Can you work these out from the model? Positions are in its coordinate system, mm. Face numbers are marked on the shaded views. A direction names the side the tool comes from. Round coordinates to 2 decimals unless told otherwise and drop trailing zeros. Write each loop counter-clockwise with the first axis right and the second up, starting at its lowest first coordinate (ties: lowest second). Pieces come first, ordered by that corner, then holes.
Q1. For the marked faces 4, 5 and 6, which set-ups out of +Z, -Z, +X, -X, +Y, -Y let a thin tool reach every point of the face, with its end or its side?
Q2. If we section it at B-B (z = 15): Please give me the cut outline in (x, y), plus the area to 3 significant figures.
Q3. If we section it at D-D (x = -14.9): Please give me the cut outline in (y, z).
Q4. Please list where these lines run through material, in increasing order: line 1 along Y through (x, z) = (0.5, 25); line 2 along Y through (x, z) = (25, 8); line 3 along Y through (x, z) = (25.5, 6).
Q5. We'd pull the mould along X, two halves only. Please class the marked faces 1, 2 and 3: +X half, -X half, draft (parallel to the pull), parting line (faces both ways), or undercut.
Q6. If we section it at C-C (y = 0): Please give me the cut outline in (x, z).
Q7. If we section it at A-A (y = -5): Please give me the cut outline in (x, z).
Q8. I'm going to push flat-ended pins straight in: pin 1 Ø22.5 at (x, z) = (10.5, 11) entering from -Y; pin 2 Ø1 at (y, z) = (-11.5, 19.5) entering from -X; pin 3 Ø2.5 at (x, y) = (11.5, 1) entering from +Z. Where does each tip first touch, or does it pass through?
from build123d import *

# Parameters (mm, degrees)
SKETCH1_W                    = 49.7
SKETCH1_H                    = 26
BOSS_EXTRUDE1_DEPTH          = 14
SKETCH2_W                    = 41.4
SKETCH2_H                    = 26
BOSS_EXTRUDE2_DEPTH          = 17
CUT_EXTRUDE1_DEPTH           = 20.5
SKETCH4_W                    = 14
SKETCH4_H                    = 26
BOSS_EXTRUDE3_DEPTH          = 7.7
BOSS_EXTRUDE5_START          = -26
SKETCH6_W                    = 8
SKETCH6_H                    = 5
BOSS_EXTRUDE5_DEPTH          = 7
SKETCH5_W                    = 7
SKETCH5_H                    = 7
BOSS_EXTRUDE6_DEPTH          = 7
SKETCH7_W                    = 4
SKETCH7_H                    = 6.5
F_3_0_3_DIAMETER_HOLE1_D     = 3
F_3_0_3_DIAMETER_HOLE1_DEPTH = 38
F_3_0_3_DIAMETER_HOLE2_D     = 3
F_3_0_3_DIAMETER_HOLE2_DEPTH = 39.1
F_3_0_3_DIAMETER_HOLE3_D     = 3
F_3_0_3_DIAMETER_HOLE3_DEPTH = 33
FILLET1_R                    = 6


with BuildPart() as part:
    # Sketch1 → Boss-Extrude1 (new body)
    with BuildSketch(Plane(origin=(0, 0, 0), x_dir=(-1, 0, 0), z_dir=(0, 0, -1))):
        with Locations((3.85, 0)):
            Rectangle(SKETCH1_W, SKETCH1_H)
    extrude(amount=-BOSS_EXTRUDE1_DEPTH)

    # Sketch2 → Boss-Extrude2 (add)
    with BuildSketch(Plane.XY.offset(14)):
        Rectangle(SKETCH2_W, SKETCH2_H)
    extrude(amount=BOSS_EXTRUDE2_DEPTH)

    # Sketch3 → Cut-Extrude1 (cut)
    with BuildSketch(Plane(origin=(0, 10.25, 0), x_dir=(1, 0, 0), z_dir=(0, 1, 0))):
        Polygon((20.7, -14), (21, -14), (21, 0), (-21, 0), (-21, -14), (-20.7, -14), (-20.7, -28.1), (20.7, -28.1), align=None)
    extrude(amount=-CUT_EXTRUDE1_DEPTH, mode=Mode.SUBTRACT)

    # Sketch4 → Boss-Extrude3 (add)
    with BuildSketch(Plane(origin=(21, 0, 0), x_dir=(0, 0, -1), z_dir=(1, 0, 0))):
        with Locations((-7, 0)):
            Rectangle(SKETCH4_W, SKETCH4_H)
    extrude(amount=BOSS_EXTRUDE3_DEPTH)

    # Sketch6 → Boss-Extrude5 (add)
    with BuildSketch(Plane(origin=(0, 13, 0), x_dir=(-1, 0, 0), z_dir=(0, 1, 0)).offset(BOSS_EXTRUDE5_START)):
        with Locations((6.4, 2.5)):
            Rectangle(SKETCH6_W, SKETCH6_H)
    extrude(amount=-BOSS_EXTRUDE5_DEPTH)

    # Sketch5 → Boss-Extrude6 (add)
    with BuildSketch(Plane.XY.offset(31)):
        with Locations((-14.9, -9.5)):
            Rectangle(SKETCH5_W, SKETCH5_H)
    extrude(amount=BOSS_EXTRUDE6_DEPTH)

    # Sketch7 → Revolve1 (revolve)
    with BuildSketch(Plane.XZ, mode=Mode.PRIVATE) as revolve1_sk:
        with Locations((12.2, 34.25)):
            Rectangle(SKETCH7_W, SKETCH7_H)
    revolve(revolve1_sk.sketch.rotate(Axis((10.2, 0, 37.5), (0, 0, -1)), 180), axis=Axis((10.2, 0, 37.5), (0, 0, -1)))

    # Ø3.0 (3) Diameter Hole1
    with Locations(Plane(origin=(0, 0, 0), x_dir=(-1, 0, 0), z_dir=(0, 0, -1))):
        with Locations((-25.5, -5), (-25.5, 5), (25.5, -5), (25.5, 5)):
            Hole(F_3_0_3_DIAMETER_HOLE1_D / 2, depth=F_3_0_3_DIAMETER_HOLE1_DEPTH)

    # Ø3.0 (3) Diameter Hole2
    with Locations(Plane.ZY.offset(10.4)):
        with Locations((2.2, -16.5)):
            Hole(F_3_0_3_DIAMETER_HOLE2_D / 2, depth=F_3_0_3_DIAMETER_HOLE2_DEPTH)

    # Ø3.0 (3) Diameter Hole3
    with Locations(Plane(origin=(0, 13, 0), x_dir=(1, 0, 0), z_dir=(0, 1, 0))):
        with Locations((-14.9, -34.5)):
            Hole(F_3_0_3_DIAMETER_HOLE3_D / 2, depth=F_3_0_3_DIAMETER_HOLE3_DEPTH)

    # Fillet1
    fillet1_edges = [part.edges().sort_by_distance(p)[0] for p in [
        (28.7, -13, 7),
        (28.7, 13, 7),
        (-28.7, 13, 7),
        (-28.7, -13, 7),
    ]]
    fillet(fillet1_edges, radius=FILLET1_R)


solid = part.part
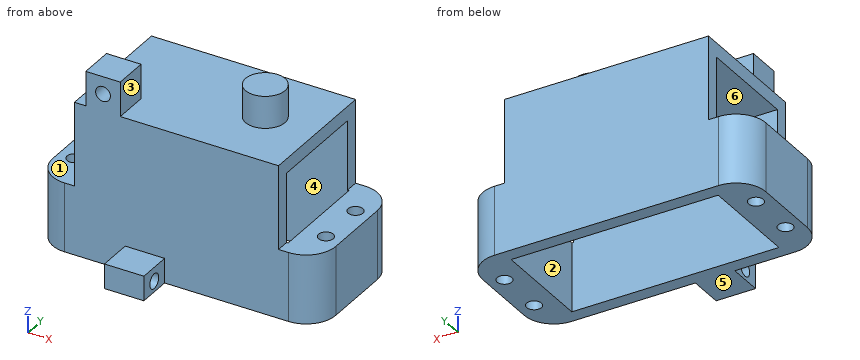
A:
1. face 4: -Z
1. face 5: -Z, +X, -X, +Y, -Y
1. face 6: -Z, +X, -X
2. outline: (-20.7, -13) - (20.7, -13) - (20.7, -10.25) - (-20.7, -10.25) - close; (-20.7, 10.25) - (20.7, 10.25) - (20.7, 13) - (-20.7, 13) - close
2. area: 228 mm2
3. outline: (-13, 0) - (-10.25, 0) - (-10.25, 28.1) - (10.25, 28.1) - (10.25, 0) - (13, 0) - (13, 31) - (-6, 31) - (-6, 33) - (-13, 33) - close; (-13, 36) - (-6, 36) - (-6, 38) - (-13, 38) - close
4. line 1: y = -13 to -10.25, 10.25 to 13
4. line 2: y = -12.54 to -6.41, -3.59 to 3.59, 6.41 to 12.54
4. line 3: y = -12.31 to -6.5, -3.5 to 3.5, 6.5 to 12.31
5. face 1: draft
5. face 2: undercut
5. face 3: +X half
6. outline: (-28.7, 0) - (-21, 0) - (-21, 14) - (-28.7, 14) - close; (-20.7, 28.1) - (20.7, 28.1) - (20.7, 31) - (14.2, 31) - (14.2, 37.5) - (6.2, 37.5) - (6.2, 31) - (-20.7, 31) - close; (21, 0) - (28.7, 0) - (28.7, 14) - (21, 14) - close
7. outline: (-28.7, 0) - (-27, 0) - (-27, 14) - (-28.7, 14) - close; (-24, 0) - (-21, 0) - (-21, 14) - (-24, 14) - close; (-20.7, 28.1) - (20.7, 28.1) - (20.7, 31) - (-20.7, 31) - close; (21, 0) - (24, 0) - (24, 14) - (21, 14) - close; (27, 0) - (28.7, 0) - (28.7, 14) - (27, 14) - close
8. pin 1: stops at y = -13
8. pin 2: stops at x = -20.7
8. pin 3: stops at z = 37.5
